Read the model definition and answer for the solid it produces. Units are mm, in the model's axes. A direction names the side the tool comes from. Give positions to 0.01 mm unless a question says otherwise; leave off trailing zeros. Write each loop counter-clockwise with the first axis right and the second up, starting at its lowest first coordinate (ties: lowest second). Pieces come first, ordered by that corner, then holes. Notation, with made-up numbers: (35.5, 74.25) -> (53.5, 74.25) arc R32 cw to (53.5, 111.25) -> close; hole circle Ø5 at (-1.5, 66.5). An arc over 180 degrees is marked (long way). Put each result on its own line as item: value. Start each with the question number.
Autodesk Inventor part; units mm, degrees
ref_plane "YZ Plane" through (0, 0, 0) normal (1, 0, 0) x (0, 1, 0)
ref_plane "XZ Plane" through (0, 0, 0) normal (0, 1, 0) x (-1, 0, 0)
ref_plane "XY Plane" through (0, 0, 0) normal (0, 0, 1) x (1, 0, 0)
sketch "Sketch1" plane through (0, 0, 0) normal (0, 1, 0) x (-1, 0, 0)
  line L0 (0, 0) -> (12, 0)
  line L1 (12, 0) -> (12, -22.8)
  line L2 (12, -22.8) -> (0, -22.8)
  line L3 (0, -22.8) -> (0, 0)
  line L4 (6, -22.8) -> (6, -11.1)
  line L5 (12, 0) -> (12, 4.65)
  line L6 (12, 4.65) -> (12.5, 4.65)
  line L7 (0, -22.8) -> (-0.5, -22.8)
  line L8 (-0.5, -22.8) -> (-0.5, -27.45)
  line L9 (12.5, 4.65) -> (-0.5, 4.65)
  line L10 (-0.5, 4.65) -> (-0.5, -27.45)
  line L11 (-0.5, -27.45) -> (12.5, -27.45)
  line L12 (12.5, -27.45) -> (12.5, 4.65)
  circle A0 centre (6, -16.95) radius 5.85
  line L13 (6, -11.1) -> (6, -8.3)
  line L14 (6, -8.3) -> (6, -11.05)
  circle A1 centre (6, -11.05) radius 2.75
  line L15 (3.25, -11.05) -> (3.25, -11.7867)
  line L16 (8.75, -11.05) -> (8.75, -11.7867)
  dimension "d0" = 22.8
  dimension "d1" = 12
  dimension "d5" = 4.65
  dimension "d6" = 0.5
  dimension "d7" = 0.5
  dimension "d8" = 4.65
  dimension "d42" = 11.7
  dimension "d43" = 2.8
  dimension "d44" = 2.75
extrude "Extrusion1" add sketch "Sketch1" along normal blind 2.8 contours L0 L1 L2 L3
extrude "Extrusion3" add sketch "Sketch1" along normal blind 7.6 contours L3 L7 L10 L9 L5 L0 | L5 L6 L12 L11 L8 L7 L2 L1
sketch "Sketch5" plane through (0, 0, 0) normal (0, -1, 0) x (1, 0, 0)
  line L0 (0.5, 4.65) -> (0.5, -27.45)
  line L1 (0.5, 4.65) -> (0.5, 0)
  line L2 (-12.5, -27.45) -> (-12.5, 4.65)
  line L3 (0.5, 0) -> (-12.5, 0)
  line L4 (-12.5, 0) -> (-12.5, -8.3)
  line L5 (-12.5, -8.3) -> (0.5, -8.3)
  line L6 (0.5, -8.3) -> (0.5, 0)
  point P0 (0, 0)
  dimension "d45" = 4.65
  dimension "d46" = 8.3
extrude "Extrusion8" add sketch "Sketch5" along normal blind 7.5
sketch "Sketch6" plane through (0, -7.5, 0) normal (0, -1, 0) x (1, 0, 0)
  line L0 (-6, -22.8) -> (-12, -22.8)
  line L1 (-6, -22.8) -> (-6, -17.2)
  circle A0 centre (-6, -17.2) radius 3.025
  line L2 (0.5, 0) -> (-12.5, 0)
  line L3 (-6, -8.3) -> (-12.5, -8.3)
  line L4 (0.5, 0) -> (-12.5, 0)
  line L5 (-12.5, 0) -> (-12.5, -8.3)
  line L6 (-12.5, -8.3) -> (0.5, -8.3)
  line L7 (0.5, -8.3) -> (0.5, 0)
  line L8 (-12.5, -8.3) -> (-7.8416, -20.9536)
  line L9 (0.5, -8.3) -> (-6, -8.3)
  line L10 (0.5, -8.3) -> (-4.2111, -21.0966)
  point P0 (0, 0)
  point P1 (-12.5, 0)
  point P2 (-8.8387, -18.2451)
  point P3 (-3.1613, -18.2451)
  dimension "d49" = 5.6
  dimension "d50" = 6.05
extrude "Extrusion9" add sketch "Sketch6" along normal blind 2
sketch "Sketch7" plane through (0, -9.5, 0) normal (0, -1, 0) x (1, 0, 0)
  arc A0 (-8.75, -11.7867) -> (-3.25, -11.7867) centre (-6, -16.95) ccw
  line L0 (-6, -22.8) -> (-6, -17.2)
  circle A1 centre (-6, -17.2) radius 3.025
  point P0 (0, 0)
  dimension "d53" = 5.6
  dimension "d54" = 6.05
extrude "Extrusion10" add sketch "Sketch7" along normal blind 4
sketch "Sketch8" plane through (-12.5, 0, 0) normal (0, 0, 1) x (1, 0, 0)
  line L0 (13, -9.5) -> (0, -9.5)
  line L1 (6.5, -9.5) -> (9, -9.5)
  line L2 (6.5, -9.5) -> (4, -9.5)
  line L3 (9, -9.5) -> (11.5, -9.5)
  line L4 (11.5, -9.5) -> (11.5, -3.5)
  line L5 (11.5, -3.5) -> (9, -3.5)
  line L6 (9, -3.5) -> (9, -9.5)
  line L7 (4, -9.5) -> (1.5, -9.5)
  line L8 (1.5, -9.5) -> (1.5, -3.5)
  line L9 (1.5, -3.5) -> (4, -3.5)
  line L10 (4, -3.5) -> (4, -9.5)
  point P0 (12.5, 0)
  point P1 (1.5, -9.5)
  dimension "d58" = 2.5
  dimension "d59" = 2.5
  dimension "d60" = 6
  dimension "d61" = 6
  dimension "d62" = 2.5
  dimension "d63" = 2.5
extrude "Extrusion11" add sketch "Sketch8" along normal blind 7
sketch "Sketch9" plane through (-11, -9.5, 0) normal (-1, 0, 0) x (0, 0, 1)
  line L0 (7, 6) -> (7, 0)
  line L1 (7, 3) -> (4, 3)
  circle A0 centre (4, 3) radius 3
  circle A1 centre (4, 3) radius 1.425
  line L2 (0, 6) -> (7, 6)
  line L3 (0, 0) -> (7, 0)
  line L4 (7, 6) -> (1.6009, 6)
  line L5 (1.6009, 6) -> (1.6009, 0)
  line L6 (1.6009, 0) -> (7, 0)
  line L7 (7, 0) -> (7, 6)
  point P0 (0, 9.5)
  point P1 (4, 6)
  point P2 (4, 0)
  dimension "d66" = 2.85
  dimension "d67" = 3
extrude "Extrusion12" cut sketch "Sketch9" against normal through all contours L0 A0 L2 | A1 | L0 L3 A0
properties part number "ServoMount"
1) A cutting plane is placed at A-A on y = -6.5. Give the vertices of the cut face in (x, z) (3 decimals), and give its area (3 significant figures).
2) For faces 1 (the face through (-6.4, -11.1, -20.2)), 2 (the face through (-1.305, -8.486, -13.203)), 3 (the face through (-6, 5, 0)), 4 (the face through (-6, 0, 2)), determine the directions among +Z, -Z, +X, -X, +Y, -Y from which every point of the face is accessible in a straight line to the end or side of a thin tool.
3) Straight lines are drawn through the part: line 1 (Y direction, x = -2.4, z = 4) (3 decimals); line 2 (X direction, y = 1.2, z = -16.95); line 3 (Z direction, x = -2, y = 3). For each, find the intervals that lie inside material, in ascending order. Write a range as [from, to].
4) A cutting plane is placed at B-B on x = -10.25. Give the vertices of the cut face in (y, z) (3 decimals), and give its area (3 significant figures).
5) Each of these flat-tipped pins is pushed along its axis until it touches: pin 1 Ø6.5 at (y, z) = (-6.5, 4) entering from +X; pin 2 Ø3 at (y, z) = (-6.5, 2.5) entering from -X; pin 3 Ø1 at (x, z) = (-6, -17.5) entering from +Y. Where does it stop, or does it pass through?
6) A cutting plane is placed at C-C on z = -17.2. Give the vertices of the cut face in (x, y) (3 decimals).
7) A cutting plane is placed at D-D on x = -7.5. Give the vertices of the cut face in (y, z).
8) For a pull along Y with two mould halves and no side action, classify faces 5 (the face through (-6, 4, -27.45)), 6 (the face through (-6, -13.5, -17)), 7 (the face through (-6, -4, -8.3)), 8 (the face through (-10, -3.5, 2)) as pulls with the +Y half, pulls with the -Y half, needs draft (parallel to the pull), parting line crosses it, or undercut.
Results found:
1. outline: (-12.5, -8.3) -> (0.5, -8.3) -> (0.5, 0) -> (-1, 0) -> (-1, 2.575) -> (-3.5, 2.575) -> (-3.5, 0) -> (-8.5, 0) -> (-8.5, 2.575) -> (-11, 2.575) -> (-11, 0) -> (-12.5, 0) -> close; (-11, 5.425) -> (-8.5, 5.425) -> (-8.5, 7) -> (-11, 7) -> close; (-3.5, 5.425) -> (-1, 5.425) -> (-1, 7) -> (-3.5, 7) -> close
1. area: 129 mm²
2. face 1: -Y
2. face 2: -Z, +X, -Y
2. face 3: +Y
2. face 4: +Z, +X, -X
3. line 1: y = [-9.5, -7.925], [-5.075, -3.5], [0, 7.6]
3. line 2: x = [-12.5, -11.85], [-0.15, 0.5]
3. line 3: z = [-27.45, -22.8], [0, 4.65]
4. outline: (-9.5, -14.412) -> (-7.5, -14.412) -> (-7.5, -8.3) -> (0, -8.3) -> (0, -12.93) -> (2.8, -12.93) -> (2.8, 0) -> (7.6, 0) -> (7.6, 4.65) -> (0, 4.65) -> (0, 0) -> (-3.5, 0) -> (-3.5, 4) arc R3 ccw to (-9.5, 4) -> close; (0, -27.45) -> (7.6, -27.45) -> (7.6, -22.8) -> (2.8, -22.8) -> (2.8, -20.97) -> (0, -20.97) -> close; hole circle Ø2.85 at (-6.5, 4)
4. area: 235 mm²
5. pin 1: stops at x = -1
5. pin 2: stops at x = -11
5. pin 3: stops at y = -7.5
6. outline: (-12.5, 0) -> (-11.845, 0) -> (-11.845, 2.8) -> (-12, 2.8) -> (-12, 7.6) -> (-12.5, 7.6) -> close; (-9.223, -9.5) -> (-9.025, -9.5) -> (-9.025, -13.5) -> (-2.975, -13.5) -> (-2.975, -9.5) -> (-2.777, -9.5) -> (-2.777, -7.5) -> (-9.223, -7.5) -> close; (-0.155, 0) -> (0.5, 0) -> (0.5, 7.6) -> (0, 7.6) -> (0, 2.8) -> (-0.155, 2.8) -> close
7. outline: (-13.5, -19.83) -> (-7.5, -19.83) -> (-7.5, -8.3) -> (0, -8.3) -> (0, -8.75) -> (2.8, -8.75) -> (2.8, 0) -> (7.6, 0) -> (7.6, 4.65) -> (0, 4.65) -> (0, 0) -> (-9.5, 0) -> (-9.5, -14.57) -> (-13.5, -14.57) -> close; (0, -27.45) -> (7.6, -27.45) -> (7.6, -22.8) -> (2.8, -22.8) -> (2.8, -22.6) -> (0, -22.6) -> close
8. face 5: needs draft
8. face 6: pulls with the -Y half
8. face 7: undercut
8. face 8: undercut
